For this review, take the finished solid that the model builds, in its own axes (mm). Coordinates: 2 decimals unless noted, no trailing zeros. Write each loop counter-clockwise with the first axis right and the second up, starting at its lowest first coordinate (ties: lowest second). Pieces come first, ordered by that corner, then holes. Notation, with made-up numbers: (27.5, 16.25) -> (66.5, 16.25) arc R8 cw to (66.5, 29.25) -> close; hole circle Ø10 at (73, 76). An arc over 180 degrees is marked (long way). Put each result on its own line as item: value. Start each with the question number.
Item 1: To check wall thickness, follow L1, parallel to Y at x = -181, z = -17.75; L2, parallel to Y at x = -181.5, z = -18.5. State the ranges of each line that lie inside material, in increasing order.
Item 2: Insertion check: P1, Ø0.6, axis at x = -190, z = -14, coming from the +Y side; P2, Ø5, axis at x = -219, z = -7, coming from the -Y side. Each pin has a flat end and moves straight along its axis. Give the tip position at first contact, or say it passes through.
Item 3: Consider section A-A on x = -206. Give the boundary of the cut face in (y, z), and give its area (3 significant figures).
```python
from build123d import *

# Parameters (mm, degrees)
SKETCH1_W           = 304.8
SKETCH1_H           = 25.4
BOSS_EXTRUDE1_DEPTH = 2.032
SKETCH2_OUTSIDE_W   = 88.572
SKETCH2_OUTSIDE_H   = 65.204
CUT_EXTRUDE2_DEPTH  = 306.863252163
SKETCH4_W           = 2.032
SKETCH4_H           = 6.604
SKETCH4_W_2         = 3.556
SKETCH4_H_2         = 2.032
SKETCH4_RX          = 3.302
SKETCH4_RY          = 3.236880332
SKETCH4_RX_2        = 2.468882323
SKETCH4_RY_2        = 2.157115795
BOSS_EXTRUDE2_DEPTH = 0.254
SKETCH5_W           = 0.254
SKETCH5_H           = 7.770905738
CUT_EXTRUDE9_DEPTH  = 0.1778


with BuildPart() as part:
    # Sketch1 → Boss-Extrude1 (new body)
    with BuildSketch(Plane(origin=(0, 0, 0), x_dir=(1, 0, 0), z_dir=(0, 1, 0))):
        with Locations((-152.4, 12.7)):
            Rectangle(SKETCH1_W, SKETCH1_H)
    extrude(amount=BOSS_EXTRUDE1_DEPTH)

    # Sketch2 outside → Cut-Extrude2 (cut, through all)
    with BuildSketch(Plane(origin=(0, 0, 0), x_dir=(0, 0, -1), z_dir=(1, 0, 0))):
        with Locations((12.7, 1.016)):
            Rectangle(SKETCH2_OUTSIDE_W, SKETCH2_OUTSIDE_H)
        Polygon((0, 0.508), (7.62, 2.032), (12.7, 2.032), (17.78, 2.032), (25.4, 0.508), (25.4, 0), (0, 0), align=None, mode=Mode.SUBTRACT)
    extrude(amount=-CUT_EXTRUDE2_DEPTH, mode=Mode.SUBTRACT)

    # Sketch4 → Boss-Extrude2 (add)
    # profile 1 of 11: a face of its own
    with BuildSketch(Plane(origin=(0, 2.032, 0), x_dir=(1, 0, 0), z_dir=(0, 1, 0))):
        with Locations((-180.848, 12.7)):
            Rectangle(SKETCH4_W, SKETCH4_H)
    # profile 2 of 11: a face of its own
    with BuildSketch(Plane(origin=(0, 2.032, 0), x_dir=(1, 0, 0), z_dir=(0, 1, 0))):
        with BuildLine():
            ThreePointArc((-179.701441188, 13.661600321), (-179.796940702, 13.568380332), (-179.832, 13.43961322))
            Line((-179.832, 13.43961322), (-179.832, 12.7))
            Line((-179.832, 12.7), (-179.832, 11.96038678))
            ThreePointArc((-179.832, 11.96038678), (-179.796940702, 11.831619668), (-179.701441188, 11.738399679))
            Line((-179.701441188, 11.738399679), (-175.49264713, 9.398))
            Line((-175.49264713, 9.398), (-174.875441188, 10.507935505))
            ThreePointArc((-174.875441188, 10.507935505), (-174.853173604, 10.701059177), (-174.973987101, 10.853363795))
            Line((-174.973987101, 10.853363795), (-177.895630596, 12.478012899))
            ThreePointArc((-177.895630596, 12.478012899), (-178.026189408, 12.7), (-177.895630596, 12.921987101))
            Line((-177.895630596, 12.921987101), (-174.973987101, 14.546636205))
            ThreePointArc((-174.973987101, 14.546636205), (-174.853173604, 14.698940823), (-174.875441188, 14.892064495))
            Line((-174.875441188, 14.892064495), (-175.49264713, 16.002))
            Line((-175.49264713, 16.002), (-179.701441188, 13.661600321))
        make_face()
    # profile 3 of 11: a face of its own
    with BuildSketch(Plane(origin=(0, 2.032, 0), x_dir=(1, 0, 0), z_dir=(0, 1, 0))):
        Polygon((-167.64, 11.684), (-167.64, 13.716), (-167.64, 16.002), (-169.672, 16.002), (-169.672, 9.398), (-167.64, 9.398), align=None)
    # profile 4 of 11: a face of its own
    with BuildSketch(Plane(origin=(0, 2.032, 0), x_dir=(1, 0, 0), z_dir=(0, 1, 0))):
        with Locations((-163.068, 12.7)):
            Rectangle(SKETCH4_W, SKETCH4_H)
    # profile 5 of 11: a face of its own
    with BuildSketch(Plane(origin=(0, 2.032, 0), x_dir=(1, 0, 0), z_dir=(0, 1, 0))):
        with Locations((-165.862, 12.7)):
            Rectangle(SKETCH4_W_2, SKETCH4_H_2)
    # profile 6 of 11: a face of its own
    with BuildSketch(Plane(origin=(0, 2.032, 0), x_dir=(1, 0, 0), z_dir=(0, 1, 0))):
        with Locations((-155.956, 12.7)):
            Rectangle(SKETCH4_W, SKETCH4_H)
    # profile 7 of 11: a face of its own
    with BuildSketch(Plane(origin=(0, 2.032, 0), x_dir=(1, 0, 0), z_dir=(0, 1, 0))):
        with BuildLine():
            ThreePointArc((-144.710582264, 12.704200751), (-144.432106164, 12.642678456), (-144.272, 12.878686819))
            Line((-144.272, 12.878686819), (-144.272, 16.002))
            Line((-144.272, 16.002), (-142.24, 16.002))
            Line((-142.24, 16.002), (-142.24, 9.398))
            Line((-142.24, 9.398), (-144.272, 9.398))
            ThreePointArc((-144.272, 9.398), (-144.372490146, 9.418723918), (-144.456582264, 9.477513932))
            Line((-144.456582264, 9.477513932), (-147.389417736, 12.58005053))
            ThreePointArc((-147.389417736, 12.58005053), (-147.667893836, 12.641572825), (-147.828, 12.405564462))
            Line((-147.828, 12.405564462), (-147.828, 9.398))
            Line((-147.828, 9.398), (-149.86, 9.398))
            Line((-149.86, 9.398), (-149.86, 16.002))
            Line((-149.86, 16.002), (-147.828, 16.002))
            Line((-147.828, 16.002), (-144.710582264, 12.704200751))
        make_face()
    # profile 8 of 11: a face of its own
    with BuildSketch(Plane(origin=(0, 2.032, 0), x_dir=(1, 0, 0), z_dir=(0, 1, 0))):
        with Locations(Location((-133.923119668, 12.7), (0, 0, -90))):
            Ellipse(SKETCH4_RX, SKETCH4_RY)
        with Locations(Location((-133.923119668, 12.7), (0, 0, 39.538825136))):
            Ellipse(SKETCH4_RX_2, SKETCH4_RY_2, mode=Mode.SUBTRACT)
    # profile 9 of 11: a face of its own
    with BuildSketch(Plane(origin=(0, 2.032, 0), x_dir=(1, 0, 0), z_dir=(0, 1, 0))):
        with Locations(Location((-122.369359004, 12.7), (0, 0, -90))):
            Ellipse(SKETCH4_RX, SKETCH4_RY)
        with Locations(Location((-122.369359004, 12.7), (0, 0, 140.461174864))):
            Ellipse(SKETCH4_RX_2, SKETCH4_RY_2, mode=Mode.SUBTRACT)
    # profile 10 of 11: a face of its own
    with BuildSketch(Plane(origin=(0, 2.032, 0), x_dir=(1, 0, 0), z_dir=(0, 1, 0))):
        with BuildLine():
            Line((-111.560968993, 11.504926098), (-110.164699128, 9.582601219))
            ThreePointArc((-110.164699128, 9.582601219), (-109.140807711, 9.563074793), (-108.572707527, 10.415129425))
            Line((-108.572707527, 10.415129425), (-110.003457223, 12.733919497))
            ThreePointArc((-110.003457223, 12.733919497), (-110.009098265, 12.991067287), (-109.787294363, 13.121297223))
            Line((-109.787294363, 13.121297223), (-109.734478672, 13.121297223))
            ThreePointArc((-109.734478672, 13.121297223), (-108.83645306, 13.493271611), (-108.464478672, 14.391297223))
            Line((-108.464478672, 14.391297223), (-108.464478672, 14.732))
            ThreePointArc((-108.464478672, 14.732), (-108.83645306, 15.630025612), (-109.734478672, 16.002))
            Line((-109.734478672, 16.002), (-111.135692822, 16.002))
            Line((-111.135692822, 16.002), (-114.052478672, 16.002))
            Line((-114.052478672, 16.002), (-114.052478672, 9.398))
            Line((-114.052478672, 9.398), (-112.020478672, 9.398))
            Line((-112.020478672, 9.398), (-112.020478672, 11.355655298))
            ThreePointArc((-112.020478672, 11.355655298), (-111.844953323, 11.597228743), (-111.560968993, 11.504926098))
        make_face()
        with BuildLine():
            Line((-110.242478672, 14.224), (-110.242478672, 14.732))
            ThreePointArc((-110.242478672, 14.732), (-110.31687355, 14.911605122), (-110.496478672, 14.986))
            Line((-110.496478672, 14.986), (-111.766478672, 14.986))
            ThreePointArc((-111.766478672, 14.986), (-111.946083795, 14.911605122), (-112.020478672, 14.732))
            Line((-112.020478672, 14.732), (-112.020478672, 14.224))
            ThreePointArc((-112.020478672, 14.224), (-111.946083795, 14.044394878), (-111.766478672, 13.97))
            Line((-111.766478672, 13.97), (-110.496478672, 13.97))
            ThreePointArc((-110.496478672, 13.97), (-110.31687355, 14.044394878), (-110.242478672, 14.224))
        make_face(mode=Mode.SUBTRACT)
    # profile 11 of 11: a face of its own
    with BuildSketch(Plane(origin=(0, 2.032, 0), x_dir=(1, 0, 0), z_dir=(0, 1, 0))):
        with BuildLine():
            ThreePointArc((-188.050459309, 11.607699185), (-188.142583121, 11.694367018), (-188.265083498, 11.725859361))
            Line((-188.265083498, 11.725859361), (-192.993173567, 11.725859361))
            ThreePointArc((-192.993173567, 11.725859361), (-193.115673944, 11.694367018), (-193.207797756, 11.607699185))
            Line((-193.207797756, 11.607699185), (-194.606359356, 9.398))
            Line((-194.606359356, 9.398), (-196.384359356, 9.398))
            Line((-196.384359356, 9.398), (-192.153128533, 16.002))
            Line((-192.153128533, 16.002), (-190.629128533, 16.002))
            Line((-190.629128533, 16.002), (-189.105128533, 16.002))
            Line((-189.105128533, 16.002), (-184.873897709, 9.398))
            Line((-184.873897709, 9.398), (-186.651897709, 9.398))
            Line((-186.651897709, 9.398), (-188.050459309, 11.607699185))
        make_face()
        with BuildLine():
            ThreePointArc((-189.551175827, 13.249859361), (-189.32866817, 13.381358984), (-189.336551639, 13.639699185))
            Line((-189.336551639, 13.639699185), (-189.792342659, 14.359839824))
            ThreePointArc((-189.792342659, 14.359839824), (-189.88446647, 14.446507657), (-190.006966847, 14.478))
            Line((-190.006966847, 14.478), (-191.251290218, 14.478))
            ThreePointArc((-191.251290218, 14.478), (-191.373790595, 14.446507657), (-191.465914407, 14.359839824))
            Line((-191.465914407, 14.359839824), (-191.921705426, 13.639699185))
            ThreePointArc((-191.921705426, 13.639699185), (-191.929588895, 13.381358984), (-191.707081238, 13.249859361))
            Line((-191.707081238, 13.249859361), (-189.551175827, 13.249859361))
        make_face(mode=Mode.SUBTRACT)
    extrude(amount=BOSS_EXTRUDE2_DEPTH)

    # Sketch5 → Cut-Extrude9 (cut)
    with BuildSketch(Plane(origin=(0, 0.488461538, 0.097692308), x_dir=(1, 0, 0), z_dir=(0, 0.9805806756909202, 0.19611613513818354))):
        with Locations((-127, 3.985079866)):
            Rectangle(SKETCH5_W, SKETCH5_H)
        with Locations((-228.6, 3.985079866)):
            Rectangle(SKETCH5_W, SKETCH5_H)
        with Locations((-203.2, 3.985079866)):
            Rectangle(SKETCH5_W, SKETCH5_H)
        with Locations((-76.2, 3.985079866)):
            Rectangle(SKETCH5_W, SKETCH5_H)
        with Locations((-177.8, 3.985079866)):
            Rectangle(SKETCH5_W, SKETCH5_H)
        with Locations((-50.8, 3.985079866)):
            Rectangle(SKETCH5_W, SKETCH5_H)
        with Locations((-25.4, 3.985079866)):
            Rectangle(SKETCH5_W, SKETCH5_H)
        with Locations((-101.6, 3.985079866)):
            Rectangle(SKETCH5_W, SKETCH5_H)
        with Locations((-152.4, 3.985079866)):
            Rectangle(SKETCH5_W, SKETCH5_H)
        with Locations((-279.4, 3.985079866)):
            Rectangle(SKETCH5_W, SKETCH5_H)
        with Locations((-254, 3.985079866)):
            Rectangle(SKETCH5_W, SKETCH5_H)
    extrude(amount=-CUT_EXTRUDE9_DEPTH, mode=Mode.SUBTRACT)


solid = part.part
```
Return value:
1. L1: 0 to 2.03
1. L2: 0 to 1.89
2. P1: y = 2.03
2. P2: y = 0
3. outline: (0, -25.4) -> (0.51, -25.4) -> (2.03, -17.78) -> (2.03, -7.62) -> (0.51, 0) -> (0, 0) -> close
3. area: 40.0 mm^2
